Can you work these out from the model? Positions are in its coordinate system, mm. A direction names the side the tool comes from. Round coordinates to 2 decimals unless told otherwise and drop trailing zeros. Order: outer loops, then holes, each group sorted by start corner. A loop starts at its lowest first (then second) coordinate and runs counter-clockwise, first axis right, second up. Notation, with made-up numbers: (19.5, 48) - (25.5, 48) arc R29 cw to (25.5, 78) - close; hole circle Ø11 at (13.5, 79.25). An arc over 180 degrees is marked (long way). Write item = value, one per line.
from build123d import *

# Parameters (mm, degrees)
CROQUIS2_W              = 10
CROQUIS2_H              = 15.834903248
CROQUIS4_R              = 15
SALIENTE_EXTRUIR1_DEPTH = 10
CROQUIS5_R              = 20
SALIENTE_EXTRUIR2_DEPTH = 10
SALIENTE_EXTRUIR5_DEPTH = 3.5
CROQUIS13_R             = 2.5
CORTAR_EXTRUIR1_DEPTH   = 10
SIMETR_A3_COPY_1_DEPTH  = 3.5
CORTAR_EXTRUIR5_DEPTH   = 10
CROQUIS21_R             = 2.4
CORTAR_EXTRUIR6_DEPTH   = 10
CROQUIS7_R              = 11
CORTAR_EXTRUIR7_DEPTH   = 10
REDONDEO1_R             = 12.5
REDONDEO2_R             = 12.5
CROQUIS22_R             = 11.5
CORTAR_EXTRUIR8_DEPTH   = 4
CROQUIS6_R              = 4
CORTAR_EXTRUIR9_DEPTH   = 8
CROQUIS23_R             = 11
CORTAR_EXTRUIR10_DEPTH  = 4
CROQUIS24_R             = 11.295388062
CROQUIS24_R_2           = 8.9
SALIENTE_EXTRUIR6_DEPTH = 0.5
SALIENTE_EXTRUIR7_START = 0.5
CROQUIS25_R             = 11.5
CROQUIS25_R_2           = 8.9
SALIENTE_EXTRUIR7_DEPTH = 0.5


with BuildPart() as part:
    # Barrer1: sweep along a path in Croquis1
    with BuildLine(Plane(origin=(0, 0, 0), x_dir=(1, 0, 0), z_dir=(0, 1, 0))) as barrer1_path:
        Line((-20, 85), (-20, 60))
        ThreePointArc((-20, 60), (-17.320508076, 50), (-10, 42.679491924))
        ThreePointArc((-10, 42.679491924), (-2.679491924, 35.358983849), (0, 25.358983849))
        Line((0, 25.358983849), (0, 0))
    # Croquis2 → Barrer1 (sweep)
    with BuildSketch(Plane.XY):
        Rectangle(CROQUIS2_W, CROQUIS2_H)
    sweep(path=barrer1_path.line)

    # Croquis4 → Saliente-Extruir1 (add)
    with BuildSketch(Plane(origin=(-15, 0, 0), x_dir=(0, 0, -1), z_dir=(1, 0, 0))):
        with Locations((85, 0)):
            Circle(CROQUIS4_R)
    extrude(amount=-SALIENTE_EXTRUIR1_DEPTH)

    # Croquis5 → Saliente-Extruir2 (add)
    with BuildSketch(Plane(origin=(5, 0, 0), x_dir=(0, 0, -1), z_dir=(1, 0, 0))):
        Circle(CROQUIS5_R)
    extrude(amount=-SALIENTE_EXTRUIR2_DEPTH)

    # Croquis12 → Saliente-Extruir5 (add)
    with BuildSketch(Plane(origin=(-15, 0, 0), x_dir=(0, 0, -1), z_dir=(1, 0, 0))):
        with BuildLine():
            ThreePointArc((90.068496439, 19.972615481), (85.068496439, 24.972615481), (80.068496439, 19.972615481))
            add(Edge.make_bspline(
                [(80.068496439, 19.972615481), (79.566731031, 15.028252388), (75.848465439, 11.643922813)],
                knots=[0, 0, 0, 1, 1, 1], degree=2))
            ThreePointArc((75.848465439, 11.643922813), (85.068496439, 14.846363713), (94.288527439, 11.643922813))
            add(Edge.make_bspline(
                [(90.068496439, 19.972615481), (90.570261847, 15.028252388), (94.288527439, 11.643922813)],
                knots=[0, 0, 0, 1, 1, 1], degree=2))
        make_face()
    saliente_extruir5 = extrude(amount=-SALIENTE_EXTRUIR5_DEPTH)

    # Simetría1: Saliente-Extruir5 across plane
    add(saliente_extruir5.mirror(Plane(origin=(-20, 0, 0), x_dir=(0, 0, 1), z_dir=(1, 0, 0))))

    # Croquis13 → Cortar-Extruir1 (cut)
    with BuildSketch(Plane(origin=(-15, 0, 0), x_dir=(0, 0, -1), z_dir=(1, 0, 0))):
        with Locations((85.068496439, 19.972615481)):
            Circle(CROQUIS13_R)
    extrude(amount=-CORTAR_EXTRUIR1_DEPTH, mode=Mode.SUBTRACT)

    # Simetría3: Saliente-Extruir5 across plane
    add(saliente_extruir5.mirror(Plane.ZX))

    # Simetría3 copy 1 sketch → Simetría3 copy 1 (add)
    with BuildSketch(Plane(origin=(-25, 0, 0), x_dir=(0, 0, -1), z_dir=(-1, 0, 0))):
        with BuildLine():
            ThreePointArc((90.068496439, 19.972615481), (85.068496439, 24.972615481), (80.068496439, 19.972615481))
            add(Edge.make_bspline(
                [(80.068496439, 19.972615481), (79.566731031, 15.028252388), (75.848465439, 11.643922813)],
                knots=[0, 0, 0, 1, 1, 1], degree=2))
            ThreePointArc((75.848465439, 11.643922813), (85.068496439, 14.846363713), (94.288527439, 11.643922813))
            add(Edge.make_bspline(
                [(90.068496439, 19.972615481), (90.570261847, 15.028252388), (94.288527439, 11.643922813)],
                knots=[0, 0, 0, 1, 1, 1], degree=2))
        make_face()
    extrude(amount=-SIMETR_A3_COPY_1_DEPTH)

    # Croquis20 → Cortar-Extruir5 (cut)
    with BuildSketch(Plane(origin=(-15, 0, 0), x_dir=(0, 0, -1), z_dir=(1, 0, 0))):
        with BuildLine():
            Line((75.916830569, 25.735778906), (95.172377376, 25.735778906))
            Line((95.172377376, 25.735778906), (95.172377376, 11.023735234))
            ThreePointArc((95.172377376, 11.023735234), (85.710763224, 14.983151058), (75.916830569, 11.93717023))
            Line((75.916830569, 11.93717023), (75.916830569, 25.735778906))
        make_face()
    extrude(amount=-CORTAR_EXTRUIR5_DEPTH, mode=Mode.SUBTRACT)

    # Croquis21 → Cortar-Extruir6 (cut)
    with BuildSketch(Plane.ZY.offset(25)):
        with Locations((-85.068496439, -19.972615481)):
            Circle(CROQUIS21_R)
    extrude(amount=-CORTAR_EXTRUIR6_DEPTH, mode=Mode.SUBTRACT)

    # Croquis7 → Cortar-Extruir7 (cut)
    with BuildSketch(Plane(origin=(5, 0, 0), x_dir=(0, 0, -1), z_dir=(1, 0, 0))):
        Circle(CROQUIS7_R)
    extrude(amount=-CORTAR_EXTRUIR7_DEPTH, mode=Mode.SUBTRACT)

    # Redondeo1
    redondeo1_edges = [part.edges().sort_by_distance(p)[0] for p in [
        (0, -7.917451624, -18.366108999),
    ]]
    fillet(redondeo1_edges, radius=REDONDEO1_R)

    # Redondeo2
    redondeo2_edges = [part.edges().sort_by_distance(p)[0] for p in [
        (0, 7.917451624, -18.366108999),
    ]]
    fillet(redondeo2_edges, radius=REDONDEO2_R)

    # Croquis22 → Cortar-Extruir8 (cut)
    with BuildSketch(Plane.ZY.offset(25)):
        with Locations((-85, 0)):
            Circle(CROQUIS22_R)
    extrude(amount=-CORTAR_EXTRUIR8_DEPTH, mode=Mode.SUBTRACT)

    # Croquis6 → Cortar-Extruir9 (cut)
    with BuildSketch(Plane(origin=(-15, 0, 0), x_dir=(0, 0, -1), z_dir=(1, 0, 0))):
        with Locations((85, 0)):
            Circle(CROQUIS6_R)
    extrude(amount=-CORTAR_EXTRUIR9_DEPTH, mode=Mode.SUBTRACT)

    # Croquis23 → Cortar-Extruir10 (cut)
    with BuildSketch(Plane(origin=(-15, 0, 0), x_dir=(0, 0, -1), z_dir=(1, 0, 0))):
        with Locations((84.704611938, 0)):
            Circle(CROQUIS23_R)
    extrude(amount=-CORTAR_EXTRUIR10_DEPTH, mode=Mode.SUBTRACT)

    # Croquis24 → Saliente-Extruir6 (add)
    with BuildSketch(Plane(origin=(-19, 0, 0), x_dir=(0, 0, -1), z_dir=(1, 0, 0))):
        with Locations((85, 0)):
            Circle(CROQUIS24_R)
        with Locations((85, 0)):
            Circle(CROQUIS24_R_2, mode=Mode.SUBTRACT)
    extrude(amount=SALIENTE_EXTRUIR6_DEPTH)

    # Croquis25 → Saliente-Extruir7 (add)
    with BuildSketch(Plane.ZY.offset(21).offset(SALIENTE_EXTRUIR7_START)):
        with Locations((-85, 0)):
            Circle(CROQUIS25_R)
        with Locations(Location((-85, 0, 0), (0, 0, 180))):
            Circle(CROQUIS25_R_2, mode=Mode.SUBTRACT)
    extrude(amount=-SALIENTE_EXTRUIR7_DEPTH)


solid = part.part
(1) If we section it at B-B (z = 0): Write out the boundary of the cut face in (x, y).
Computed:
outline = (-5, -20) - (5, -20) - (5, -11) - (-5, -11) - close; (-5, 11) - (5, 11) - (5, 20) - (-5, 20) - close
(2) Thinking about a two-plate mould opening in Y: for faces 4 (the face through (-23.27, 0.51, -96.49)), 5 (the face through (0.07, -9.106, -19.967)), 6 (the face through (-21.5, -7, -79)), 7 (the face through (-15, -7, -75)), which applies, +Y half, -Y half, draft (parallel to the pull), parting line (faces both ways), or undercut?
Computed:
face_4 = undercut
face_5 = -Y half
face_6 = undercut
face_7 = draft
(3) On a 3-axis mill with a long thin cutter (end or side, diameter ignored), from which of +Z, -Z, +X, -X, +Y, -Y can I reach the whole of each face in a straight line? I mean faces 1 (the face through (-21, -2, -81)), 2 (the face through (-5, -9, -7)), 3 (the face through (-14, -7.917, -48)). Say none if no direction works.
Computed:
face_1 = -X
face_2 = +Z, -X, +Y, -Y
face_3 = +X, -X, -Y
(4) If we section it at A-A (y = 0): State how many separate pieces and enclosed holes the cut face has, plus the area to 3 significant figures.
Computed:
separate_pieces = 3
enclosed_holes = 0
area = 861 mm^2
(5) Will these pins go through, and if not, where does the flat tip stop? P1, Ø1.5, axis at x = -16.5, y = -7.5, coming from the +Z side; P2, Ø6, axis at y = -19.97, z = -85.07, coming from the +X side; P3, Ø15, axis at x = -6.5, z = -42.5, coming from the -Y side.
Computed:
P1 = -40.59
P2 = -15
P3 = -7.92
(6) If I drill on line 1 (Y direction, x = -22.2, z = -85); line 2 (Y direction, x = -2, z = 0); line 3 (X direction, y = -16, z = 9), over which ranges is the centre line in solid material (lowest first)? Write a range as from..to.
Computed:
line_1 = -24.97..-22.37, -17.57..-11.5, 11.5..15
line_2 = -20..-11, 11..20
line_3 = -5..5
